Build history of the part. All positions in model axes, mm. A direction names the side the tool comes from. Give positions to 0.01 mm unless a question says otherwise; leave off trailing zeros. Order: outer loops, then holes, each group sorted by start corner. A loop starts at its lowest first (then second) coordinate and runs counter-clockwise, first axis right, second up. Notation, with made-up numbers: M -39,17 L 15,17 A24 ccw 15,42 Z; hole C -18.75,17 d1. An arc over 180 degrees is marked long. One line per item, written item: value.
Autodesk Fusion 360 part; units mm, degrees
sketch "Esboço1" plane through (0, 0, 0) normal (0, 1, 0) x (1, 0, 0)
  line L0 (0, 0) -> (20, 0)
  line L1 (0, 0) -> (-20, 0)
  line L2 (-20, 0) -> (-20, 120)
  line L3 (-20, 120) -> (20, 120)
  line L4 (20, 120) -> (20, 0)
  dimension "d1" = 20
  dimension "d2" = 20
  dimension "d3" = 120
  dimension "d4" = 40
extrude "Extrusão1" add sketch "Esboço1" along normal blind 28
sketch "Esboço2" plane through (0, 0, 0) normal (0, 0, 1) x (1, 0, 0)
  line L0 (-20, 0) -> (20, 0)
  line L1 (20, 0) -> (20, 28)
  line L2 (20, 28) -> (-20, 28)
  line L3 (-20, 28) -> (-20, 0)
  line L4 (0, 0) -> (0, 28) construction
  line L5 (0, 14) -> (0, 27)
  line L6 (0, 27) -> (18, 27)
  line L7 (18, 14) -> (18, 27)
  line L8 (18, 14) -> (18, 1)
  line L9 (18, 1) -> (0, 1)
  line L10 (-18, 1) -> (0, 1)
  line L11 (-18, 14) -> (-18, 1)
  line L12 (-18, 14) -> (-18, 27)
  line L13 (0, 27) -> (-18, 27)
  dimension "d7" = 18
  dimension "d9" = 13
extrude "Extrusão2" cut sketch "Esboço2" against normal blind 115 contours L6 L7 L8 L9 L10 L11 L12 L13
sketch "Esboço3" plane through (0, 28, 0) normal (0, 1, 0) x (-1, 0, 0)
  line L0 (20, 0) -> (-20, 0)
  line L1 (-20, 0) -> (-20, -120)
  line L2 (-20, -120) -> (20, -120)
  line L3 (20, -120) -> (20, 0)
  line L4 (0, 0) -> (10, 0)
  line L5 (0, 0) -> (-10, 0)
  line L6 (-8, -20) -> (8, -20)
  line L7 (-8, -2) -> (-8, -20)
  line L8 (8, -2) -> (8, -20)
  line L9 (10, 0) -> (7.8787, -2.1213)
  line L10 (-10, 0) -> (-7.8787, -2.1213)
  dimension "d13" = 10
  dimension "d14" = 10
  dimension "d19" = 135
  dimension "d20" = 3
  dimension "d22" = 3
extrude "Extrusão3" cut sketch "Esboço3" against normal blind 40 contours L0 L4 L5 L6 L7 L8 L9 L10
sketch "Esboço4" plane through (20, 0, 0) normal (1, 0, 0) x (0, 0, -1)
  line L0 (0, 0) -> (120, 0)
  line L1 (120, 0) -> (120, 28)
  line L2 (120, 28) -> (0, 28)
  line L3 (0, 28) -> (0, 0)
  line L4 (120, 14) -> (120, 14.9)
  line L5 (120, 14) -> (120, 13.1)
  line L6 (120, 13.1) -> (0, 13.1)
  line L7 (120, 14.9) -> (0, 14.9)
  line L8 (0, 14.9) -> (0, 13.1)
  dimension "d25" = 0.9
  dimension "d26" = 0.9
extrude "Extrusão4" cut sketch "Esboço4" against normal blind 1 contours L1 L3 L4 L5 L6 L7 L8
sketch "Esboço5" plane through (-20, 0, 0) normal (-1, 0, 0) x (0, 0, 1)
  line L0 (-120, 0) -> (0, 0)
  line L1 (0, 0) -> (0, 28)
  line L2 (0, 28) -> (-120, 28)
  line L3 (-120, 28) -> (-120, 0)
  line L4 (0, 13.1) -> (0, 14.9)
  line L5 (0, 14.9) -> (-120, 14.9)
  line L6 (0, 13.1) -> (-120, 13.1)
  line L7 (-120, 13.1) -> (-120, 13.3204)
  line L8 (-120, 14.9) -> (-120, 13.1)
  line L9 (-120, 13.1) -> (-120, 14.9)
  dimension "d30" = 1.8
extrude "Extrusão5" cut sketch "Esboço5" against normal blind 1 contours L1 L3 L4 L5 L6 L7 L8 L9
sketch "Esboço6" plane through (0, 0, -120) normal (0, 0, -1) x (-1, 0, 0)
  line L0 (20, 13.1) -> (19, 13.1)
  line L1 (19, 13.1) -> (19, 14.9)
  line L2 (19, 14.9) -> (20, 14.9)
  line L3 (20, 14.9) -> (20, 28)
  line L4 (20, 28) -> (-20, 28)
  line L5 (-20, 28) -> (-20, 14.9)
  line L6 (-20, 14.9) -> (-19, 14.9)
  line L7 (-19, 14.9) -> (-19, 13.1)
  line L8 (-19, 13.1) -> (-20, 13.1)
  line L9 (-20, 13.1) -> (-20, 0)
  line L10 (-20, 0) -> (20, 0)
  line L11 (20, 0) -> (20, 13.1)
  line L12 (-19, 14.9) -> (19, 14.9)
  line L13 (19, 13.1) -> (-19, 13.1)
extrude "Extrusão6" cut sketch "Esboço6" against normal blind 1 contours L1 L7 L12 L13
equation "d9 = ( 26 / 2 ) * 1 mm"
1) Saw through at B-B, the plane x = 2. Write the cut outline in (y, z), then the cut area to 3 significant figures.
Check values:
outline: M 0,-120 L 13.1,-120 L 13.1,-119 L 14.9,-119 L 14.9,-120 L 28,-120 L 28,-20 L 27,-20 L 27,-115 L 1,-115 L 1,-20 L 0,-20 Z
area: 328 mm^2
2) Mould opens along X. For faces 1 (the face through (20, 21, -61)), 2 (the face through (0, 0, -61)), 3 (the face through (-9, 0.5, -1)) say: released by +X, released by -X, zero draft, split by the parting line, or undercut.
Check values:
face 1: released by +X
face 2: zero draft
face 3: undercut
3) Saw through at A-A, the plane z = -13. Write the cut outline in (x, y).
Check values:
outline: M -20,0 L -8,0 L -8,1 L -18,1 L -18,27 L -8,27 L -8,28 L -20,28 L -20,14.9 L -19,14.9 L -19,13.1 L -20,13.1 Z; M 8,0 L 20,0 L 20,13.1 L 19,13.1 L 19,14.9 L 20,14.9 L 20,28 L 8,28 L 8,27 L 18,27 L 18,1 L 8,1 Z
4) Saw through at D-D, the plane z = -103. Write the cut outline in (x, y), then the cut area to 3 significant figures.
Check values:
outline: M -20,0 L 20,0 L 20,13.1 L 19,13.1 L 19,14.9 L 20,14.9 L 20,28 L -20,28 L -20,14.9 L -19,14.9 L -19,13.1 L -20,13.1 Z; hole M -18,1 L 18,1 L 18,27 L -18,27 Z
area: 180 mm^2
5) Drill centre lines: probe 1 along X at (y, z) = (16.75, -110); probe 2 along Y at (x, z) = (-11.5, -62.5); probe 3 along Z at (x, y) = (-4, 15). Where is each one in solid material? Low to high. Write a range as from..to.
Check values:
probe 1: -20..-18, 18..20
probe 2: 0..1, 27..28
probe 3: -120..-115
6) Pin check, flat tips, straight feed: pin 1 (0.8 mm diameter, centred on x = 1.5, y = 0.5, fed in from +Z); pin 2 (13 mm diameter, centred on x = 4, y = 19.5, fed in from +Z); pin 3 (0.9 mm diameter, centred on y = 14, z = -37.5, fed in from +X). Stop position of each tip, or through.
Check values:
pin 1: z = -20
pin 2: z = -115
pin 3: x = 19
7) Saw through at C-C, the plane y = 22.5. Write the cut outline in (x, z), then the cut area to 3 significant figures.
Check values:
outline: M -20,-120 L 20,-120 L 20,0 L 18,0 L 18,-115 L -18,-115 L -18,0 L -20,0 Z
area: 660 mm^2
8) Tool access for faces 4 (the face through (-9, 27.5, -1)), 5 (the face through (20, 6, -61)), 6 (the face through (0, 14, -115)): list every direction of +Z, -Z, +X, -X, +Y, -Y with a clear straight run to the whole face (end or side of a thin tool).
Check values:
face 4: +Z, +Y, -Y
face 5: +Z, -Z, +X, +Y, -Y
face 6: +Z
